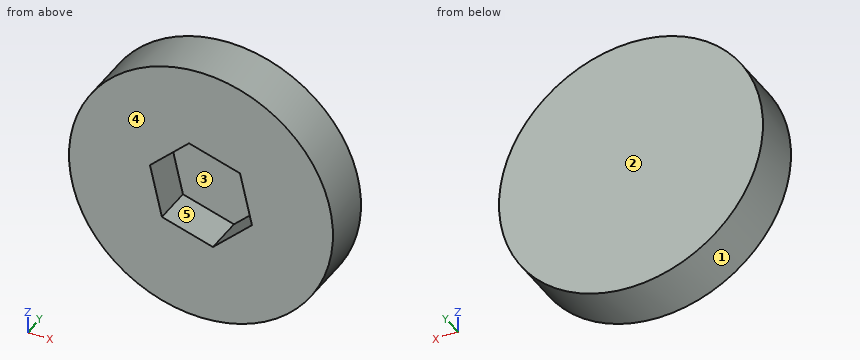
from build123d import *

# Parameters (mm, degrees)
SKETCH1_R           = 10
BOSS_EXTRUDE1_DEPTH = 3
CUT_EXTRUDE2_DEPTH  = 15.456832295
SKETCH3_R           = 10
BOSS_EXTRUDE2_DEPTH = 1


with BuildPart() as part:
    # Sketch1 → Boss-Extrude1 (new body)
    with BuildSketch(Plane(origin=(0, 0, 0), x_dir=(1, 0, 0), z_dir=(0, 1, 0))):
        with Locations(Location((0, 0, 0), (0, 0, 270))):
            Circle(SKETCH1_R)
    extrude(amount=BOSS_EXTRUDE1_DEPTH)

    # Sketch2 → Cut-Extrude2 (cut, through all)
    with BuildSketch(Plane(origin=(0, 3, 0), x_dir=(1, 0, 0), z_dir=(0, 1, 0))):
        Polygon((2.958730451, -2.753043307), (3.863570667, 1.18581408), (0.904840216, 3.938857387), (-2.958730451, 2.753043307), (-3.863570667, -1.18581408), (-0.904840216, -3.938857387), align=None)
    extrude(amount=-CUT_EXTRUDE2_DEPTH, mode=Mode.SUBTRACT)

    # Sketch3 → Boss-Extrude2 (add)
    with BuildSketch(Plane(origin=(0, 3, 0), x_dir=(1, 0, 0), z_dir=(0, 1, 0))):
        with Locations(Location((0, 0, 0), (0, 0, 270))):
            Circle(SKETCH3_R)
    extrude(amount=BOSS_EXTRUDE2_DEPTH)


solid = part.part
The listing builds one solid part. Answer for the finished solid, in the listing's coordinates (mm). Face numbers are marked on the shaded views. A direction names the side the tool comes from. Round coordinates to 2 decimals unless told otherwise and drop trailing zeros. Order: outer loops, then holes, each group sorted by start corner. A loop starts at its lowest first (then second) coordinate and runs counter-clockwise, first axis right, second up. Notation, with made-up numbers: (16, 37.25) -> (56, 37.25) arc R19 cw to (56, 59.25) -> close; hole circle Ø2 at (-26, 59). An arc over 180 degrees is marked (long way). One line per item, written item: value.
Item 1: Straight lines are drawn through the part: L1, parallel to X at y = 0.5, z = 0; L2, parallel to Y at x = 1, z = 1.25; L3, parallel to Z at x = -2, y = 2.2. For each, find the intervals that lie inside material, in ascending order.
Taken from the geometry:
L1: x = -10 to -3.59, 3.59 to 10
L2: y = 3 to 4
L3: z = -9.8 to -3.05, 2.92 to 9.8
Item 2: Find section C-C, the plane x = 0. Give the vertices of the cut face in (y, z).
Taken from the geometry:
outline: (0, -10) -> (4, -10) -> (4, 10) -> (0, 10) -> (0, 3.66) -> (3, 3.66) -> (3, -3.66) -> (0, -3.66) -> close
Item 3: For a pull along X with two mould halves and no side action, classify the marked faces 1, 2 and 3 as released by +X, released by -X, zero draft, split by the parting line, or undercut.
Taken from the geometry:
face 1: split by the parting line
face 2: zero draft
face 3: undercut
Item 4: Find section D-D, the plane z = 8. Give the vertices of the cut face in (x, y), then the cut area to 3 significant figures.
Taken from the geometry:
outline: (-6, 0) -> (6, 0) -> (6, 4) -> (-6, 4) -> close
area: 48.0 mm2
Item 5: Given P1, Ø4, axis at x = 0, z = 0.5, coming from the -Y side, flat-ended and moving along its own axis, determine where the tip first touches the part or whether it passes through.
Taken from the geometry:
P1: stops at y = 3
Item 6: Find section A-A, the plane y = 2.5. Give the vertices of the cut face in (x, z), then the cut area to 3 significant figures.
Taken from the geometry:
outline: circle Ø20 at (0, 0); hole (-3.86, 1.19) -> (-2.96, -2.75) -> (0.9, -3.94) -> (3.86, -1.19) -> (2.96, 2.75) -> (-0.9, 3.94) -> close
area: 272 mm2
Item 7: Find section B-B, the plane z = 0. Give the vertices of the cut face in (x, y), then the cut area to 3 significant figures.
Taken from the geometry:
outline: (-10, 0) -> (-3.59, 0) -> (-3.59, 3) -> (3.59, 3) -> (3.59, 0) -> (10, 0) -> (10, 4) -> (-10, 4) -> close
area: 58.5 mm2
Item 8: For the marked faces 4 and 5, determine the directions among +Z, -Z, +X, -X, +Y, -Y from which every point of the face is accessible in a straight line to the end or side of a thin tool.
Taken from the geometry:
face 4: +Z, -Z, +X, -X, -Y
face 5: -Y
